from build123d import *

# Parameters (mm, degrees)
SKETCH1_W                                           = 125
SKETCH1_H                                           = 125
EXTRUDE1_DEPTH                                      = 16
CBORE_FOR_M4_HEX_SOCKET_HEAD_CAP_SCREW1_D           = 4.5
CBORE_FOR_M4_HEX_SOCKET_HEAD_CAP_SCREW1_CBORE_D     = 8
CBORE_FOR_M4_HEX_SOCKET_HEAD_CAP_SCREW1_CBORE_DEPTH = 4.4
CBORE_FOR_M6_HEX_SOCKET_HEAD_CAP_SCREW1_D           = 6.6
CBORE_FOR_M6_HEX_SOCKET_HEAD_CAP_SCREW1_CBORE_D     = 11
CBORE_FOR_M6_HEX_SOCKET_HEAD_CAP_SCREW1_CBORE_DEPTH = 6.4
M6_TAPPED_HOLE1_D                                   = 5
M4_TAPPED_HOLE1_D                                   = 3.3
M4_TAPPED_HOLE1_DEPTH                               = 11.5
M4_TAPPED_HOLE1_TIP                                 = 0.991420021


with BuildPart() as part:
    # Sketch1 → Extrude1 (new body)
    with BuildSketch(Plane(origin=(0, 0, 0), x_dir=(1, 0, 0), z_dir=(0, 1, 0))):
        Rectangle(SKETCH1_W, SKETCH1_H)
    extrude(amount=EXTRUDE1_DEPTH)

    # CBORE for M4 Hex Socket Head Cap Screw1 (through all)
    with Locations(Plane(origin=(0, 16, 0), x_dir=(1, 0, 0), z_dir=(0, 1, 0))):
        with Locations((-49, 56), (-23, 56), (-49, 30), (-23, 30), (23, 30), (49, 30), (23, 56), (49, 56), (49, -56), (23, -56), (49, -30), (23, -30), (-23, -56), (-23, -30), (-49, -30), (-49, -56)):
            CounterBoreHole(CBORE_FOR_M4_HEX_SOCKET_HEAD_CAP_SCREW1_D / 2, CBORE_FOR_M4_HEX_SOCKET_HEAD_CAP_SCREW1_CBORE_D / 2, CBORE_FOR_M4_HEX_SOCKET_HEAD_CAP_SCREW1_CBORE_DEPTH)

    # CBORE for M6 Hex Socket Head Cap Screw1 (through all)
    with Locations(Plane(origin=(0, 16, 0), x_dir=(1, 0, 0), z_dir=(0, 1, 0))):
        with Locations((27, 17.5), (27, -17.5)):
            CounterBoreHole(CBORE_FOR_M6_HEX_SOCKET_HEAD_CAP_SCREW1_D / 2, CBORE_FOR_M6_HEX_SOCKET_HEAD_CAP_SCREW1_CBORE_D / 2, CBORE_FOR_M6_HEX_SOCKET_HEAD_CAP_SCREW1_CBORE_DEPTH)

    # M6 Tapped Hole1 (through all)
    with Locations(Plane(origin=(0, 16, 0), x_dir=(1, 0, 0), z_dir=(0, 1, 0))):
        with Locations((-50, 45), (50, 45), (50, -45), (-50, -45), (0, 0)):
            Hole(M6_TAPPED_HOLE1_D / 2)

    # M4 Tapped Hole1
    with Locations(Plane(origin=(0, 0, -62.5), x_dir=(-1, 0, 0), z_dir=(0, 0, -1))):
        with Locations((36, 7.5), (24, 7.5)):
            Hole(M4_TAPPED_HOLE1_D / 2, depth=M4_TAPPED_HOLE1_DEPTH)
            with Locations((0, 0, -(M4_TAPPED_HOLE1_DEPTH + M4_TAPPED_HOLE1_TIP / 2))):  # 118° drill point
                Cone(0, M4_TAPPED_HOLE1_D / 2, M4_TAPPED_HOLE1_TIP, mode=Mode.SUBTRACT)


solid = part.part
For this review, take the finished solid that the model builds, in its own axes (mm). A direction names the side the tool comes from. Give positions to 0.01 mm unless a question says otherwise; leave off trailing zeros. Loops run counter-clockwise (first coordinate to the right, second up) from the corner with the lowest first, then second, coordinate; pieces in that order, holes last. Notation, with made-up numbers: M 48,-2 L 78,-2 A11 cw 78,6 Z; hole C 21,9 d6. An arc over 180 degrees is marked long. Answer as a JSON object with one key per item and string values. Group by question number.
Q1. For probe 1 along X at (y, z) = (12.75, -45); probe 2 along X at (y, z) = (13.65, -30); probe 3 along X at (y, z) = (7.5, 30), list the stretches that pass through material, from the lowest coordinate up. Write a range as [from, to].
Q2. Add section B-B on y = 13.75. Give the number of separate pieces and of enclosed holes in the cut face, and give its area (3 significant figures).
Q3. Insertion check: P1, Ø6.5, axis at x = 23, z = 56, coming from the +Y side; P2, Ø3.5, axis at x = -49, z = -30, coming from the -Y side; P3, Ø5.5, axis at x = 26.5, z = -15, coming from the +Y side. Each pin has a flat end and moves straight along its axis. Give the tip position at first contact, or say it passes through.
Q4. Mouldability with a two-part tool opening along Z and no side actions: class faces 3 (the conical face through (-24.3, 7.6, -50.2)), 4 (the flat face through (-15, 0, -1)), 5 (the flat face through (-1, 8, 62.5)), 6 (the cylindrical face through (23.95, 4.73, -16.24)) as +Z half, -Z half, draft (parallel to the pull), parting line (faces both ways), or undercut.
Q5. Add section C-C on z = 17.5. Give the boundary of the cut face in (x, y).
Q6. Tool access review of faces 1 (the flat face through (27, 9.6, -14)), 2 (the cylindrical face through (51.248, 5.719, 29.901)): name each direction out of +Z, -Z, +X, -X, +Y, -Y from which nothing blocks a thin tool from reaching the whole face with its end or side.
Q7. Add section A-A on x = 0. Give the boundary of the cut face in (y, z).
Checked values:
{
 "1": {"probe 1": "[-62.5, -52.5], [-47.5, 47.5], [52.5, 62.5]", "probe 2": "[-62.5, -53], [-45, -27], [-19, 19], [27, 45], [53, 62.5]", "probe 3": "[-62.5, -51.25], [-46.75, -25.25], [-20.75, 20.75], [25.25, 46.75], [51.25, 62.5]"},
 "2": {"separate pieces": "1", "enclosed holes": "23", "area": "14,500 mm²"},
 "3": {"P1": "y = 11.6", "P2": "through", "P3": "y = 9.6"},
 "4": {"face 3": "-Z half", "face 4": "draft", "face 5": "+Z half", "face 6": "undercut"},
 "5": {"outline": "M -62.5,0 L 23.7,0 L 23.7,9.6 L 21.5,9.6 L 21.5,16 L -62.5,16 Z; M 30.3,0 L 62.5,0 L 62.5,16 L 32.5,16 L 32.5,9.6 L 30.3,9.6 Z"},
 "6": {"face 1": "+Y", "face 2": "+Y, -Y"},
 "7": {"outline": "M 0,-62.5 L 16,-62.5 L 16,-2.5 L 0,-2.5 Z; M 0,2.5 L 16,2.5 L 16,62.5 L 0,62.5 Z"}
}
